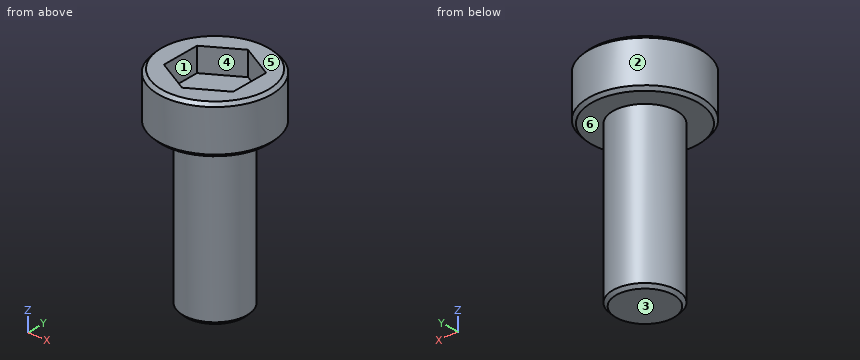
from build123d import *

# Parameters (mm, degrees)
SKETCH_1_R          = 2
EXTRUDE_1_DEPTH     = 16
SKETCH_2_R          = 3.52854217
EXTRUDE_3_DEPTH     = 3
CUT_EXTRUDE_2_DEPTH = 1.5
CHAMFER_1_SIZE      = 0.2
CHAMFER_2_SIZE      = 0.2
SKETCH_4_R          = 2
CUT_EXTRUDE_3_DEPTH = 6
CHAMFER_3_SIZE      = 0.2


with BuildPart() as part:
    # 草图1 → 凸台-拉伸1 (new body)
    with BuildSketch(Plane.XY):
        Circle(SKETCH_1_R)
    extrude(amount=EXTRUDE_1_DEPTH)

    # 草图2 → 凸台-拉伸3 (add)
    with BuildSketch(Plane.XY.offset(16)):
        Circle(SKETCH_2_R)
    extrude(amount=EXTRUDE_3_DEPTH)

    # 草图3 → 切除-拉伸2 (cut)
    with BuildSketch(Plane.XY.offset(19)):
        Polygon((0, 2.497687594), (-2.163060907, 1.248843797), (-2.163060907, -1.248843797), (0, -2.497687594), (2.163060907, -1.248843797), (2.163060907, 1.248843797), align=None)
    extrude(amount=-CUT_EXTRUDE_2_DEPTH, mode=Mode.SUBTRACT)

    # 倒角1
    chamfer_1_edges = [part.edges().sort_by_distance(p)[0] for p in [
        (-2, 0, 0),
    ]]
    chamfer(chamfer_1_edges, length=CHAMFER_1_SIZE)

    # 倒角2
    chamfer_2_edges = [part.edges().sort_by_distance(p)[0] for p in [
        (-3.52854217, 0, 16),
        (-3.52854217, 0, 19),
    ]]
    chamfer(chamfer_2_edges, length=CHAMFER_2_SIZE)

    # 草图4 → 切除-拉伸3 (cut)
    with BuildSketch(Plane(origin=(0, 0, 0), x_dir=(-1, 0, 0), z_dir=(0, 0, -1))):
        Circle(SKETCH_4_R)
    extrude(amount=-CUT_EXTRUDE_3_DEPTH, mode=Mode.SUBTRACT)

    # 倒角3
    chamfer_3_edges = [part.edges().sort_by_distance(p)[0] for p in [
        (-2, 0, 6),
    ]]
    chamfer(chamfer_3_edges, length=CHAMFER_3_SIZE)


solid = part.part
Read the model definition and answer for the solid it produces. Units are mm, in the model's axes. Face numbers are marked on the shaded views. A direction names the side the tool comes from. Coordinates: 2 decimals unless noted, no trailing zeros. Loops run counter-clockwise (first coordinate to the right, second up) from the corner with the lowest first, then second, coordinate; pieces in that order, holes last. Notation, with made-up numbers: (-23, -5) -> (-4, -5) arc R17 ccw to (-4, 15) -> close; hole circle Ø7 at (70, -7). An arc over 180 degrees is marked (long way). Answer in a Markdown table with one row per item.
Item 1: For the marked faces 4, 5 and 6, determine the directions among +Z, -Z, +X, -X, +Y, -Y from which every point of the face is accessible in a straight line to the end or side of a thin tool.
Returned:
| item | result |
|---|---|
| face 4 | +Z |
| face 5 | +Z, +X, -X, +Y, -Y |
| face 6 | -Z |
Item 2: For a pull along Y with two mould halves and no side action, classify the marked faces 1, 2 and 3 as released by +Y, released by -Y, zero draft, split by the parting line, or undercut.
Returned:
| item | result |
|---|---|
| face 1 | undercut |
| face 2 | split by the parting line |
| face 3 | zero draft |
Item 3: Each of these flat-tipped pins is pushed along its axis until it touches: P1, Ø1.3, axis at x = -1, y = -0.5, coming from the +Z side; P2, Ø3, axis at y = -1, z = 13.5, coming from the +X side; P3, Ø1, axis at x = 1, z = 8.5, coming from the -Y side; P4, Ø1.5, axis at x = -1, y = 2, coming from the -Z side. Where does it stop, or does it pass through?
Returned:
| item | result |
|---|---|
| P1 | stops at z = 17.5 |
| P2 | stops at x = 2 |
| P3 | stops at y = -1.94 |
| P4 | stops at z = 6 |
Item 4: Straight lines are drawn through the part: line 1 along Z through (x, y) = (-3, -1); line 2 along Z through (x, y) = (0, -0.5); line 3 along X through (y, z) = (-1, 18.25). For each, find the intervals that lie inside material, in ascending order. Write a range as [from, to].
Returned:
| item | result |
|---|---|
| line 1 | z = [16, 19] |
| line 2 | z = [6, 17.5] |
| line 3 | x = [-3.38, -2.16], [2.16, 3.38] |
Item 5: A cutting plane is placed at A-A on y = 0. Determine the outline of the cut face in (x, z).
Returned:
| item | result |
|---|---|
| outline | (-3.53, 16.2) -> (-3.33, 16) -> (-2, 16) -> (-2, 6.2) -> (-1.8, 6) -> (1.8, 6) -> (2, 6.2) -> (2, 16) -> (3.33, 16) -> (3.53, 16.2) -> (3.53, 18.8) -> (3.33, 19) -> (2.16, 19) -> (2.16, 17.5) -> (-2.16, 17.5) -> (-2.16, 19) -> (-3.33, 19) -> (-3.53, 18.8) -> close |
